```python
from build123d import *

# Parameters (mm, degrees)
SKETCH_2_R      = 27
SKETCH_2_R_2    = 6.2
SKETCH_2_R_3    = 1.5
EXTRUDE_1_DEPTH = 3


with BuildPart() as part:
    # 草图2 → 凸台-拉伸1 (new body)
    with BuildSketch(Plane.XY):
        Circle(SKETCH_2_R)
        Circle(SKETCH_2_R_2, mode=Mode.SUBTRACT)
        with Locations((22.51, 0)):
            Circle(SKETCH_2_R_3, mode=Mode.SUBTRACT)
        with Locations((11.255, -19.494231839)):
            Circle(SKETCH_2_R_3, mode=Mode.SUBTRACT)
        with Locations((-11.255, -19.494231839)):
            Circle(SKETCH_2_R_3, mode=Mode.SUBTRACT)
        with Locations((-22.51, 0)):
            Circle(SKETCH_2_R_3, mode=Mode.SUBTRACT)
        with Locations((-11.255, 19.494231839)):
            Circle(SKETCH_2_R_3, mode=Mode.SUBTRACT)
        with Locations((11.255, 19.494231839)):
            Circle(SKETCH_2_R_3, mode=Mode.SUBTRACT)
    extrude(amount=EXTRUDE_1_DEPTH)


solid = part.part
```
The model under review builds one solid part; all positions refer to its coordinate system, in mm. Round coordinates to 2 decimals unless told otherwise and drop trailing zeros. Order: outer loops, then holes, each group sorted by start corner. A loop starts at its lowest first (then second) coordinate and runs counter-clockwise, first axis right, second up.
(1) Take a section at C-C, the plane x = 11. State the section outline as (y, z) points.
Working result:
outline: (-24.66, 0) - (-20.97, 0) - (-20.97, 3) - (-24.66, 3) - close; (-18.02, 0) - (18.02, 0) - (18.02, 3) - (-18.02, 3) - close; (20.97, 0) - (24.66, 0) - (24.66, 3) - (20.97, 3) - close
(2) Mouldability with a two-part tool opening along X and no side actions: class faces 1 (the face through (-5.85, -26.36, 1.48)), 2 (the face through (-12.36, 20.51, 1.48)), 3 (the face through (-6.4, 0.4, 3)), 4 (the face through (21.01, 0.07, 1.48)) as released by +X, released by -X, zero draft, split by the parting line, or undercut.
Working result:
face 1: split by the parting line
face 2: undercut
face 3: zero draft
face 4: undercut
(3) Wall thickness on L1, parallel to Y at x = 0, z = 1; L2, parallel to Y at x = -11.5, z = 0.7; L3, parallel to X at y = 18.5, z = 0.75: over which ranges is each line inside the solid? List them lowest first.
Working result:
L1: y = -27 to -6.2, 6.2 to 27
L2: y = -24.43 to -20.97, -18.01 to 18.01, 20.97 to 24.43
L3: x = -19.67 to -12.38, -10.13 to 10.13, 12.38 to 19.67
(4) For P1, Ø1, axis at x = 1, y = 4, coming from the -Z side; P2, Ø1.5, axis at x = 12.5, z = 2, coming from the -Y side; P3, Ø1.5, axis at y = 17, z = 0.5, coming from the -X side, all flat-tipped, find the tip position at first contact; note any pin that passes through.
Working result:
P1: passes through
P2: stops at y = -24.31
P3: stops at x = -21.56
(5) Take a section at B-B, the plane x = 0. State the section outline as (y, z) points.
Working result:
outline: (-27, 0) - (-6.2, 0) - (-6.2, 3) - (-27, 3) - close; (6.2, 0) - (27, 0) - (27, 3) - (6.2, 3) - close
(6) Take a section at D-D, the plane z = 1.35. State the section outline as (x, y) points (3 decimals).
Working result:
outline: circle Ø54 at (0, 0); hole circle Ø3 at (-22.51, 0); hole circle Ø3 at (-11.255, -19.494); hole circle Ø3 at (-11.255, 19.494); hole circle Ø12.4 at (0, 0); hole circle Ø3 at (11.255, -19.494); hole circle Ø3 at (11.255, 19.494); hole circle Ø3 at (22.51, 0)
(7) Take a section at A-A, the plane y = 0. State the section outline as (x, z) points.
Working result:
outline: (-27, 0) - (-24.01, 0) - (-24.01, 3) - (-27, 3) - close; (-21.01, 0) - (-6.2, 0) - (-6.2, 3) - (-21.01, 3) - close; (6.2, 0) - (21.01, 0) - (21.01, 3) - (6.2, 3) - close; (24.01, 0) - (27, 0) - (27, 3) - (24.01, 3) - close
